```python
from build123d import *

# Parameters (mm, degrees)
F0_W      = 70.4
F0_H      = 48.4
F2_DEPTH  = 27
F3_T      = -2
F4_R      = 1.5
F1_R      = 2
F1_R_2    = 3.75
F5_DEPTH  = 25
F6_DEPTH  = 8
F1_W      = 35.2
F1_H      = 19.2
F7_DEPTH  = 25
F9_DEPTH  = 25
F11_DEPTH = 25


# Not quite as in the source:
# - a feature names something its author has since deleted; it is built from what else it names


with BuildPart() as f2:
    # F0 (on Top) → F2 (new body)
    with BuildSketch(Plane.XY):
        Rectangle(F0_W, F0_H)
    extrude(amount=F2_DEPTH)

    # F3
    f3_openings = [f2.faces().sort_by_distance(p)[0] for p in [
        (0, 0, 27),
    ]]
    offset(amount=F3_T, openings=f3_openings)

    # F4
    f4_edges = [f2.edges().sort_by_distance(p)[0] for p in [
        (-35.2, 24.2, 13.5),
        (-35.2, -24.2, 13.5),
        (-35.2, 0, 0),
        (0, 24.2, 0),
        (0, -24.2, 0),
        (35.2, 0, 0),
        (35.2, -24.2, 13.5),
        (35.2, 24.2, 13.5),
    ]]
    fillet(f4_edges, radius=F4_R)

    # F1 (on Top) → F5 (cut)
    with BuildSketch(Plane.XY):
        with Locations((-22.1, -13.1)):
            Circle(F1_R)
        with Locations((-22.1, 2.4)):
            Circle(F1_R_2)
    extrude(amount=F5_DEPTH, mode=Mode.SUBTRACT)

    # F1 (on Top) → F6 (join)
    with BuildSketch(Plane.XY):
        with BuildLine():
            Line((27, 17.5), (26, 17.5))
            ThreePointArc((26, 17.5), (26.732233047, 15.732233047), (28.5, 15))
            Line((28.5, 15), (28.5, 16))
            ThreePointArc((28.5, 16), (27.4393398282, 16.4393398282), (27, 17.5))
        make_face()
        with BuildLine():
            ThreePointArc((31, 17.5), (28.5, 20), (26, 17.5))
            Line((26, 17.5), (27, 17.5))
            ThreePointArc((27, 17.5), (28.5, 19), (30, 17.5))
            ThreePointArc((30, 17.5), (29.5606601718, 16.4393398282), (28.5, 16))
            Line((28.5, 16), (28.5, 15))
            ThreePointArc((28.5, 15), (30.267766953, 15.732233047), (31, 17.5))
        make_face()
        with BuildLine():
            Line((28.5, -16), (28.5, -15))
            ThreePointArc((28.5, -15), (26.732233047, -15.732233047), (26, -17.5))
            Line((26, -17.5), (27, -17.5))
            ThreePointArc((27, -17.5), (27.4393398282, -16.4393398282), (28.5, -16))
        make_face()
        with BuildLine():
            ThreePointArc((31, -17.5), (30.267766953, -15.732233047), (28.5, -15))
            Line((28.5, -15), (28.5, -16))
            ThreePointArc((28.5, -16), (29.5606601718, -16.4393398282), (30, -17.5))
            ThreePointArc((30, -17.5), (28.5, -19), (27, -17.5))
            Line((27, -17.5), (26, -17.5))
            ThreePointArc((26, -17.5), (28.5, -20), (31, -17.5))
        make_face()
        with BuildLine():
            Line((-28.5, -16), (-28.5, -15))
            ThreePointArc((-28.5, -15), (-30.267766953, -19.267766953), (-26, -17.5))
            Line((-26, -17.5), (-27, -17.5))
            ThreePointArc((-27, -17.5), (-29.5606601718, -18.5606601718), (-28.5, -16))
        make_face()
        with BuildLine():
            ThreePointArc((-26, -17.5), (-26.732233047, -15.732233047), (-28.5, -15))
            Line((-28.5, -15), (-28.5, -16))
            ThreePointArc((-28.5, -16), (-27.4393398282, -16.4393398282), (-27, -17.5))
            Line((-27, -17.5), (-26, -17.5))
        make_face()
        with BuildLine():
            Line((-27, 17.5), (-26, 17.5))
            ThreePointArc((-26, 17.5), (-30.267766953, 19.267766953), (-28.5, 15))
            Line((-28.5, 15), (-28.5, 16))
            ThreePointArc((-28.5, 16), (-29.5606601718, 18.5606601718), (-27, 17.5))
        make_face()
        with BuildLine():
            ThreePointArc((-28.5, 15), (-26.732233047, 15.732233047), (-26, 17.5))
            Line((-26, 17.5), (-27, 17.5))
            ThreePointArc((-27, 17.5), (-27.4393398282, 16.4393398282), (-28.5, 16))
            Line((-28.5, 16), (-28.5, 15))
        make_face()
    extrude(amount=F6_DEPTH)

    # F1 (on Top) → F7 (cut)
    with BuildSketch(Plane.XY):
        with Locations((8.5, 3.5)):
            Rectangle(F1_W, F1_H)
    extrude(amount=F7_DEPTH, mode=Mode.SUBTRACT)

    # F8 (on face) → F9 (join)
    with BuildSketch(Plane.XY.offset(2)):
        with BuildLine():
            ThreePointArc((-33.2, 19.6), (-31.3615223689, 20.3615223689), (-30.6, 22.2))
            Line((-30.6, 22.2), (-31.7, 22.2))
            ThreePointArc((-31.7, 22.2), (-32.1393398282, 21.1393398282), (-33.2, 20.7))
            Line((-33.2, 20.7), (-33.2, 19.6))
        make_face()
        with BuildLine():
            Line((31.7, 22.2), (30.6, 22.2))
            ThreePointArc((30.6, 22.2), (31.3615223689, 20.3615223689), (33.2, 19.6))
            Line((33.2, 19.6), (33.2, 20.7))
            ThreePointArc((33.2, 20.7), (32.1393398282, 21.1393398282), (31.7, 22.2))
        make_face()
        with BuildLine():
            Line((33.2, -20.7), (33.2, -19.6))
            ThreePointArc((33.2, -19.6), (31.3615223689, -20.3615223689), (30.6, -22.2))
            Line((30.6, -22.2), (31.7, -22.2))
            ThreePointArc((31.7, -22.2), (32.1393398282, -21.1393398282), (33.2, -20.7))
        make_face()
        with BuildLine():
            ThreePointArc((-30, -21.6), (-30.9875484503, -19.5603921946), (-33.2, -19.0701778719))
            Line((-33.2, -19.0701778719), (-33.2, -20.2252272915))
            ThreePointArc((-33.2, -20.2252272915), (-31.7784161637, -20.3450099602), (-31.1, -21.6))
            ThreePointArc((-31.1, -21.6), (-31.1316405306, -21.9064644655), (-31.2252272915, -22.2))
            Line((-31.2252272915, -22.2), (-30.0701778719, -22.2))
            ThreePointArc((-30.0701778719, -22.2), (-30.0176040647, -21.9020450851), (-30, -21.6))
        make_face()
    extrude(amount=F9_DEPTH)

    # F10 (on face) → F11 (cut)
    with BuildSketch(Plane.XY.offset(27)):
        with BuildLine():
            Line((-33.2, 22.2), (-31.7, 22.2))
            ThreePointArc((-31.7, 22.2), (-34.2606601718, 23.2606601718), (-33.2, 20.7))
            Line((-33.2, 20.7), (-33.2, 22.2))
        make_face()
        with BuildLine():
            ThreePointArc((-33.2, 20.7), (-32.1393398282, 21.1393398282), (-31.7, 22.2))
            Line((-31.7, 22.2), (-33.2, 22.2))
            Line((-33.2, 22.2), (-33.2, 20.7))
        make_face()
        with BuildLine():
            ThreePointArc((33.2, 20.7), (34.2606601718, 21.1393398282), (34.7, 22.2))
            ThreePointArc((34.7, 22.2), (33.2, 23.7), (31.7, 22.2))
            Line((31.7, 22.2), (33.2, 22.2))
            Line((33.2, 22.2), (33.2, 20.7))
        make_face()
        with BuildLine():
            Line((33.2, 22.2), (31.7, 22.2))
            ThreePointArc((31.7, 22.2), (32.1393398282, 21.1393398282), (33.2, 20.7))
            Line((33.2, 20.7), (33.2, 22.2))
        make_face()
        with BuildLine():
            ThreePointArc((31.7, -22.2), (33.2, -23.7), (34.7, -22.2))
            ThreePointArc((34.7, -22.2), (34.2606601718, -21.1393398282), (33.2, -20.7))
            Line((33.2, -20.7), (33.2, -22.2))
            Line((33.2, -22.2), (31.7, -22.2))
        make_face()
        with BuildLine():
            Line((-33.2, -22.2), (-33.2, -20.2252272915))
            ThreePointArc((-33.2, -20.2252272915), (-33.6606601718, -22.6606601718), (-31.2252272915, -22.2))
            Line((-31.2252272915, -22.2), (-33.2, -22.2))
        make_face()
    extrude(amount=-F11_DEPTH, mode=Mode.SUBTRACT)


solid = f2.part
```
Source: CAD feature listing. Evaluate the final solid. Frame: model axes, mm. A direction names the side the tool comes from. Round coordinates to 2 decimals unless told otherwise and drop trailing zeros. Write each loop counter-clockwise with the first axis right and the second up, starting at its lowest first coordinate (ties: lowest second). Pieces come first, ordered by that corner, then holes. Notation, with made-up numbers: M 57.25,43.5 L 100.25,43.5 A20 ccw 100.25,57.5 Z; hole C 51,0 d2. An arc over 180 degrees is marked long. Answer as a JSON object with one key per item and string values. Group by question number.
(1) Section query B-B on y = 7. Output: boundary loops of the cut face in (x, z).
(2) Reachability of faces 5 (the flat face through (30, -19, 8)), 6 (the flat face through (26.1, 3, 1)), 7 (the flat face through (35.2, 0, 14)) from +Z, -Z, +X, -X, +Y, -Y: full face, straight path, thin tool, end or side. Return the list, or none.
(3) First-contact query: pin 1 (3.5 mm diameter, centred on x = -29, y = -17, fed in from +Z); pin 2 (2.5 mm diameter, centred on x = -28.5, y = 17.5, fed in from +Z). Flat tips, straight axial feed; report the tip coordinate or a pass-through.
(4) Ray query, line 1 (X direction, y = -17.5, z = 6.4); line 2 (Y direction, x = -22.1, z = 1.6); line 3 (X direction, y = 2.4, z = 1.5). Return the intervals inside material, ascending. Write a range as [from, to].
(5) Section query A-A on z = 25. Output: boundary loops of the cut face in (x, y), then the cut area to 3 significant figures.
(6) Mould query, pull axis Y, two halves, no side actions, for faces 1 (the flat face through (33.2, 0, 14)), 2 (the flat face through (33, -22, 2)), 3 (the cylindrical face through (-34.77, 0.32, 0.45)), 4 (the cylindrical face through (0.47, -23.77, 0.45)). Classes: +Y half, -Y half, draft (parallel to the pull), parting line (faces both ways), or undercut.
(7) Section query D-D on x = -22.5. Output: boundary loops of the cut face in (y, z), then the cut area to 3 significant figures.
(8) Section query C-C on x = -1.5. Output: boundary loops of the cut face in (y, z), then the cut area to 3 significant figures.
Computed values:
{
 "1": {"outline": "M -35.2,1.5 A1.5 ccw -33.7,0 L -9.1,0 L -9.1,2 L -33.2,2 L -33.2,27 L -35.2,27 Z; M 26.1,0 L 33.7,0 A1.5 ccw 35.2,1.5 L 35.2,27 L 33.2,27 L 33.2,2 L 26.1,2 Z"},
 "2": {"face 5": "+Z", "face 6": "+Z, -Z", "face 7": "+Z, -Z, +X, +Y, -Y"},
 "3": {"pin 1": "z = 8", "pin 2": "z = 2"},
 "4": {"line 1": "[-35.2, -33.2], [-31, -30], [-27, -26], [26, 27], [30, 31], [33.2, 35.2]", "line 2": "[-24.2, -15.1], [-11.1, -1.35], [6.15, 24.2]", "line 3": "[-35.2, -25.85], [-18.35, -9.1], [26.1, 35.2]"},
 "5": {"outline": "M -35.2,-22.7 A1.5 ccw -33.7,-24.2 L 33.7,-24.2 A1.5 ccw 35.2,-22.7 L 35.2,22.7 A1.5 ccw 33.7,24.2 L -33.7,24.2 A1.5 ccw -35.2,22.7 Z; hole C -33.2,22.2 d3; hole C -32.6,-21.6 d3; hole M -33.2,-19.07 A2.6 cw -30.07,-22.2 L 30.6,-22.2 A2.6 cw 33.2,-19.6 L 33.2,19.6 A2.6 cw 30.6,22.2 L -30.6,22.2 A2.6 cw -33.2,19.6 Z; hole C 33.2,-22.2 d3; hole C 33.2,22.2 d3", "area": "454 mm^2"},
 "6": {"face 1": "undercut", "face 2": "undercut", "face 3": "draft", "face 4": "-Y half"},
 "7": {"outline": "M -24.2,1.5 A1.5 ccw -22.7,0 L -15.06,0 L -15.06,2 L -22.2,2 L -22.2,27 L -24.2,27 Z; M -11.14,0 L -1.33,0 L -1.33,2 L -11.14,2 Z; M 6.13,0 L 22.7,0 A1.5 ccw 24.2,1.5 L 24.2,27 L 22.2,27 L 22.2,2 L 6.13,2 Z", "area": "173 mm^2"},
 "8": {"outline": "M -24.2,1.5 A1.5 ccw -22.7,0 L -6.1,0 L -6.1,2 L -22.2,2 L -22.2,27 L -24.2,27 Z; M 13.1,0 L 22.7,0 A1.5 ccw 24.2,1.5 L 24.2,27 L 22.2,27 L 22.2,2 L 13.1,2 Z", "area": "157 mm^2"}
}
